For this review, take the finished solid that the model builds, in its own axes (mm). A direction names the side the tool comes from. Round coordinates to 2 decimals unless told otherwise and drop trailing zeros. Order: outer loops, then holes, each group sorted by start corner. A loop starts at its lowest first (then second) coordinate and runs counter-clockwise, first axis right, second up. Notation, with made-up numbers: M 72,66 L 93,66 A19 cw 93,74 Z; hole C 23.5,78 d2. An arc over 180 degrees is marked long. Put each result on its own line as item: value.
from build123d import *

# Parameters (mm, degrees)
F0_R     = 15.5321
F0_R_2   = 2.38125
F1_DEPTH = 42.3672
F3_DEPTH = 42.3672
F4_COUNT = 12
F4_ANGLE = 330


with BuildPart() as f1:
    # F0 (on Top) → F1 (new body)
    with BuildSketch(Plane.XY):
        Circle(F0_R)
        Circle(F0_R_2, mode=Mode.SUBTRACT)
    extrude(amount=F1_DEPTH)

    # F2 (on face) → F3 (cut, through all)
    with BuildSketch(Plane.XY.offset(42.3672)):
        with BuildLine():
            Line((-0.3108154952, 12.3531904437), (-0.3108154952, 2.3608780761))
            Line((-0.3108154952, 2.3608780761), (0, 2.3608780761))
            Line((0, 2.3608780761), (0.3108154952, 2.3608780761))
            Line((0.3108154952, 2.3608780761), (0.3108154952, 12.3531904437))
            ThreePointArc((0.3108154952, 12.3531904437), (0, 12.3571), (-0.3108154952, 12.3531904437))
        make_face()
    f3 = extrude(amount=-F3_DEPTH, mode=Mode.SUBTRACT)

    # F4: F3 ×12 about axis
    f4_axis = Axis((0, 0, 0), (0, 0, 1))
    for i in range(1, F4_COUNT):
        add(f3.rotate(f4_axis, i * F4_ANGLE / (F4_COUNT - 1)), mode=Mode.SUBTRACT)


solid = f1.part
(1) Add section A-A on y = -5. Give the boundary of the cut face in (x, z).
A:
outline: M -14.71,0 L -9.28,0 L -9.28,42.37 L -14.71,42.37 Z; M -8.04,0 L -3.25,0 L -3.25,42.37 L -8.04,42.37 Z; M -2.53,0 L -0.31,0 L -0.31,42.37 L -2.53,42.37 Z; M 0.31,0 L 2.53,0 L 2.53,42.37 L 0.31,42.37 Z; M 3.25,0 L 8.04,0 L 8.04,42.37 L 3.25,42.37 Z; M 9.28,0 L 14.71,0 L 14.71,42.37 L 9.28,42.37 Z
(2) To check wall thickness, follow L1, parallel to Y at x = 3, z = 19; L2, parallel to X at y = 3.5, z = 6; L3, parallel to Y at x = -7.5, z = 27. State the ranges of each line that lie inside material, in increasing order.
A:
L1: y = -15.24 to -5.82, -4.57 to -2.09, -1.37 to -0.31, 0.31 to 1.37, 2.09 to 4.57, 5.82 to 15.24
L2: x = -15.13 to -6.68, -5.44 to -2.38, -1.66 to -0.31, 0.31 to 1.66, 2.38 to 5.44, 6.68 to 15.13
L3: y = -13.6 to -4.69, -3.97 to -0.31, 0.31 to 3.97, 4.69 to 13.6
(3) Insertion check: pin 1 Ø5 at (y, z) = (-8.5, 23.5) entering from -X; pin 2 Ø12 at (x, z) = (8, 31) entering from -Y; pin 3 Ø11 at (x, z) = (7, 30) entering from -Y. Each pin has a flat end and moves straight along its axis. Give the tip position at first contact, or say it passes through.
A:
pin 1: stops at x = -14.33
pin 2: stops at y = -15.4
pin 3: stops at y = -15.46
(4) For faces 1 (the face through (3, -3, 42.367)), 2 (the face through (-3.983, 6.277, 21.48)), list the 3-axis set-ups (+Z, -Z, +X, -X, +Y, -Y) from which the entire face can be reached by the end or side of a thin tool; tool diameter is ignored.
A:
face 1: +Z, +X, -X, +Y, -Y
face 2: +Z, -Z
